```python
from build123d import *

# Parameters (mm, degrees)
F0_W     = 38.1
F0_H     = 88.9
F1_DEPTH = 1416.05
F2_W     = 19.05
F2_H     = 63.5
F3_DEPTH = 101.6
F4_W     = 19.05
F4_H     = 63.5
F5_DEPTH = 101.6
F6_W     = 88.9
F6_H     = 19.05
F7_DEPTH = 19.05


with BuildPart() as f1:
    # F0 (on Right) → F1 (new body)
    with BuildSketch(Plane.YZ):
        Rectangle(F0_W, F0_H)
    extrude(amount=F1_DEPTH)

    # F2 (on face) → F3 (join)
    with BuildSketch(Plane.YZ.offset(1416.05)):
        Rectangle(F2_W, F2_H)
    extrude(amount=F3_DEPTH)

    # F4 (on face) → F5 (join)
    with BuildSketch(Plane(origin=(0, 0, 0), x_dir=(0, -1, 0), z_dir=(-1, 0, 0))):
        Rectangle(F4_W, F4_H)
    extrude(amount=F5_DEPTH)

    # F6 (on face) → F7 (cut)
    with BuildSketch(Plane.XY.offset(44.45)):
        with Locations((78.994, 0)):
            Rectangle(F6_W, F6_H)
        with Locations((218.694, 0)):
            Rectangle(F6_W, F6_H)
        with Locations((358.394, 0)):
            Rectangle(F6_W, F6_H)
        with Locations((498.094, 0)):
            Rectangle(F6_W, F6_H)
        with Locations((637.794, 0)):
            Rectangle(F6_W, F6_H)
        with Locations((777.494, 0)):
            Rectangle(F6_W, F6_H)
        with Locations((917.194, 0)):
            Rectangle(F6_W, F6_H)
        with Locations((1056.894, 0)):
            Rectangle(F6_W, F6_H)
        with Locations((1196.594, 0)):
            Rectangle(F6_W, F6_H)
        with Locations((1336.294, 0)):
            Rectangle(F6_W, F6_H)
    extrude(amount=-F7_DEPTH, mode=Mode.SUBTRACT)


solid = f1.part
```
Source: CAD feature listing. Evaluate the final solid. Frame: model axes, mm. A direction names the side the tool comes from. Round coordinates to 2 decimals unless told otherwise and drop trailing zeros. Order: outer loops, then holes, each group sorted by start corner. A loop starts at its lowest first (then second) coordinate and runs counter-clockwise, first axis right, second up. Notation, with made-up numbers: (-18, 73) -> (-1, 73) arc R24 cw to (-1, 85) -> close; hole circle Ø2 at (-39, 33.5). An arc over 180 degrees is marked (long way). One line per item, written item: value. Start each with the question number.
Q1. Material intervals for probe 1 along Y at (x, z) = (660.5, 34.5) (3 decimals); probe 2 along X at (y, z) = (-12.5, -15.5); probe 3 along Z at (x, y) = (1293, -9), sorted ascending.
Q2. Pin query (flat end, axial travel): pin 1 (4 mm diameter, centred on y = 13, z = 23.5, fed in from +X); pin 2 (5.5 mm diameter, centred on x = 73.5, y = -4.5, fed in from +Z); pin 3 (5.5 mm diameter, centred on y = 4.5, z = 35, fed in from -X). Return the tip coordinate at first contact, or that it passes through.
Q3. Section query A-A (x = 74). Return the cut outline in (y, z) (3 decimals).
Q4. Access query for faces 1 (the flat face through (1466, 9.525, 0)), 2 (the flat face through (1466, -9.525, 0)), 3 (the flat face through (-50, -9.525, 0)), 4 (the flat face through (-50, 9.525, 0)). Directions: +Z, -Z, +X, -X, +Y, -Y. A direction counts if a zero-diameter tool reaches every point of the face in a straight line with its end or side. Return the directions, or none.
Findings below:
1. probe 1: -19.05 to -9.525, 9.525 to 19.05
1. probe 2: 0 to 1416.05
1. probe 3: -44.45 to 25.4
2. pin 1: x = 1416.05
2. pin 2: z = 25.4
2. pin 3: x = 0
3. outline: (-19.05, -44.45) -> (19.05, -44.45) -> (19.05, 44.45) -> (9.525, 44.45) -> (9.525, 25.4) -> (-9.525, 25.4) -> (-9.525, 44.45) -> (-19.05, 44.45) -> close
4. face 1: +Z, -Z, +X, +Y
4. face 2: +Z, -Z, +X, -Y
4. face 3: +Z, -Z, -X, -Y
4. face 4: +Z, -Z, -X, +Y
